Can you work these out from the model? Positions are in its coordinate system, mm. Coordinates: 2 decimals unless noted, no trailing zeros. Order: outer loops, then holes, each group sorted by start corner. A loop starts at its lowest first (then second) coordinate and runs counter-clockwise, first axis right, second up. Notation, with made-up numbers: M -2.5,69 L 44.5,69 A35 cw 44.5,103 Z; hole C 51.5,41 d10. An arc over 180 degrees is marked long. Answer as a JSON object with one key per item and string values.
from build123d import *

# Parameters (mm, degrees)
SKETCH1_R           = 0.5
BOSS_EXTRUDE1_DEPTH = 0.762
FILLET1_R           = 2.54


with BuildPart() as part:
    # Sketch1 → Boss-Extrude1 (new body)
    with BuildSketch(Plane.XY):
        with BuildLine():
            Line((-0.508, 13.0175), (-1.30175, 13.81125))
            Line((-1.30175, 13.81125), (0, 17.78))
            Line((0, 17.78), (1.30175, 13.81125))
            Line((1.30175, 13.81125), (0.508, 13.0175))
            Line((0.508, 13.0175), (0.508, 1.504025349))
            ThreePointArc((0.508, 1.504025349), (1.5875, 0), (0.508, -1.504025349))
            Line((0.508, -1.504025349), (0.508, -17.78))
            Line((0.508, -17.78), (-0.508, -17.78))
            Line((-0.508, -17.78), (-0.508, -1.504025349))
            ThreePointArc((-0.508, -1.504025349), (-1.5875, 0), (-0.508, 1.504025349))
            Line((-0.508, 1.504025349), (-0.508, 13.0175))
        make_face()
        Circle(SKETCH1_R, mode=Mode.SUBTRACT)
    extrude(amount=BOSS_EXTRUDE1_DEPTH)

    # Fillet1
    fillet1_edges = [part.edges().sort_by_distance(p)[0] for p in [
        (0.508, -1.504025349, 0.381),
        (-0.508, -1.504025349, 0.381),
        (-0.508, 1.504025349, 0.381),
        (0.508, 1.504025349, 0.381),
    ]]
    fillet(fillet1_edges, radius=FILLET1_R)


solid = part.part
Item 1: Please list where these lines run through material, in increasing order: line 1 (X direction, y = -7, z = 0.65); line 2 (Y direction, x = -1.4, z = 0.3); line 3 (X direction, y = 1.5, z = 0.2).
Answers follow:
{"line 1": "x = -0.51 to 0.51", "line 2": "y = -0.75 to 0.75", "line 3": "x = -0.86 to 0.86"}
Item 2: I want a section at D-D, the plane y = 11.5. Write out the boundary of the cut face in (x, z), plus the area to 3 significant figures.
Answers follow:
{"outline": "M -0.51,0 L 0.51,0 L 0.51,0.76 L -0.51,0.76 Z", "area": "0.774 mm^2"}
Item 3: If we mould it in two halves opening along X, with no side actions, what happens to faces 1 (the flat face through (-1, 0, 0.762)), 2 (the flat face through (-0.66, 15.77, 0.38)), 3 (the cylindrical face through (-0.108, -0.488, 0.376))? For each: pulls with the +X half, pulls with the -X half, needs draft (parallel to the pull), parting line crosses it, or undercut.
Answers follow:
{"face 1": "needs draft", "face 2": "pulls with the -X half", "face 3": "undercut"}
Item 4: I want a section at A-A, the plane y = 0. Write out the boundary of the cut face in (x, z), plus the area to 3 significant figures.
Answers follow:
{"outline": "M -1.59,0 L -0.5,0 L -0.5,0.76 L -1.59,0.76 Z; M 0.5,0 L 1.59,0 L 1.59,0.76 L 0.5,0.76 Z", "area": "1.66 mm^2"}
Item 5: I want a section at C-C, the plane x = -0.8. Write out the boundary of the cut face in (y, z), plus the area to 3 significant figures.
Answers follow:
{"outline": "M -1.6,0 L 1.6,0 L 1.6,0.76 L -1.6,0.76 Z; M 13.31,0 L 15.34,0 L 15.34,0.76 L 13.31,0.76 Z", "area": "3.99 mm^2"}
Item 6: I want a section at B-B, the plane z = 0.35. Write out the boundary of the cut face in (x, y) (1 decimal).
Answers follow:
{"outline": "M -1.3,13.8 L -0.5,13 L -0.5,2.8 A2.5 cw -1.2,1.1 A1.6 ccw -1.2,-1.1 A2.5 cw -0.5,-2.8 L -0.5,-17.8 L 0.5,-17.8 L 0.5,-2.8 A2.5 cw 1.2,-1.1 A1.6 ccw 1.2,1.1 A2.5 cw 0.5,2.8 L 0.5,13 L 1.3,13.8 L 0,17.8 Z; hole C 0,0 d1"}
